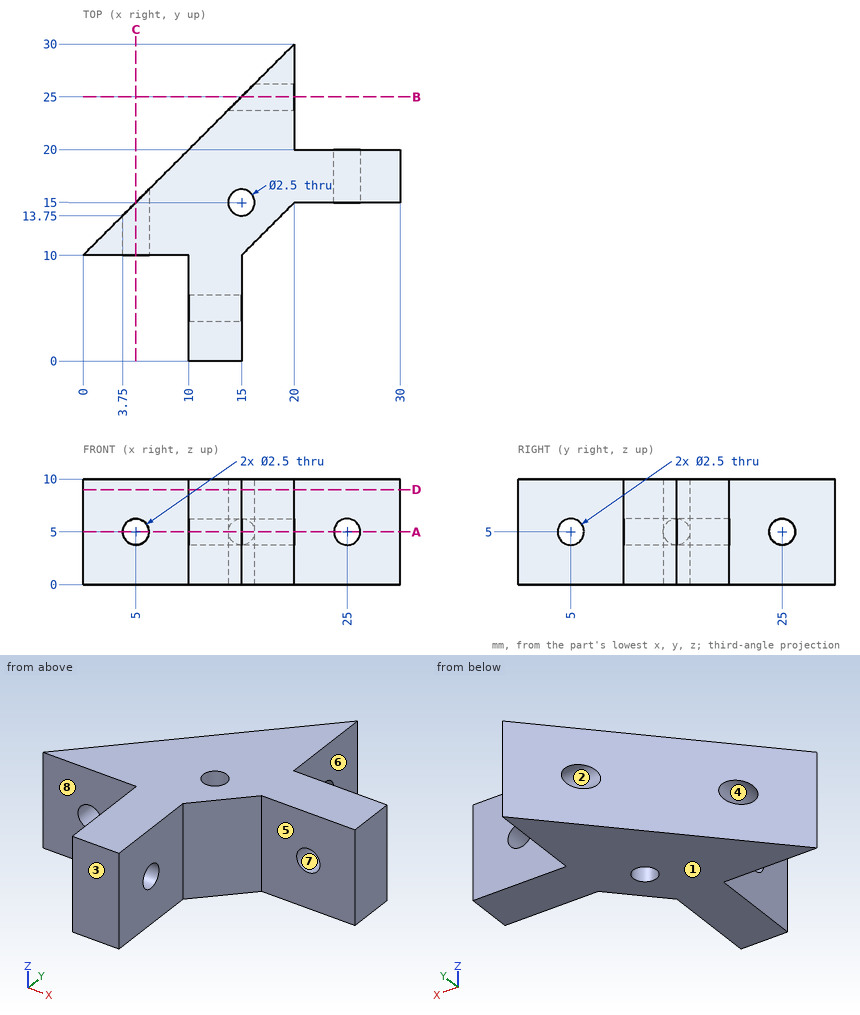
Part print with two shaded views. Sizes in mm from the minimum x, y, z corner. A direction names the side the tool comes from. Coordinates: 2 decimals unless noted, no trailing zeros. Write each loop counter-clockwise with the first axis right and the second up, starting at its lowest first coordinate (ties: lowest second). Pieces come first, ordered by that corner, then holes. Notation, with made-up numbers: (16.25, 55) - (63.25, 55) arc R12 cw to (63.25, 71) - close; hole circle Ø10 at (32.25, -18.75). An arc over 180 degrees is marked (long way). Put each result on its own line as item: value.
1. Band-saw the part on B-B (y = 25). Write the cut outline in (x, z).
Final values:
outline: (15, 0) - (20, 0) - (20, 3.75) - (15, 3.75) - close; (15, 6.25) - (20, 6.25) - (20, 10) - (15, 10) - close
2. Band-saw the part on C-C (x = 5). Write the cut outline in (y, z), then the cut area to 3 significant figures.
Final values:
outline: (10, 0) - (15, 0) - (15, 3.75) - (10, 3.75) - close; (10, 6.25) - (15, 6.25) - (15, 10) - (10, 10) - close
area: 37.5 mm²
3. Flat gauge pins, fed straight in: pin 1 Ø3 at (y, z) = (26.5, 6) entering from +X; pin 2 Ø5 at (x, z) = (25, 4) entering from -Y; pin 3 Ø6 at (x, z) = (20, 3) entering from -Y; pin 4 Ø6 at (x, y) = (4, 20) entering from +Z. Where does each tip first touch, or does it go through?
Final values:
pin 1: stops at x = 20
pin 2: stops at y = 15
pin 3: stops at y = 12
pin 4: passes through
4. Band-saw the part on A-A (z = 5). Write the cut outline in (x, y).
Final values:
outline: (0, 10) - (3.75, 10) - (3.75, 13.75) - close; (6.25, 10) - (10, 10) - (10, 6.25) - (15, 6.25) - (15, 10) - (20, 15) - (23.75, 15) - (23.75, 20) - (20, 20) - (20, 23.75) - (13.75, 23.75) - (6.25, 16.25) - close; (10, 0) - (15, 0) - (15, 3.75) - (10, 3.75) - close; (16.25, 26.25) - (20, 26.25) - (20, 30) - close; (26.25, 15) - (30, 15) - (30, 20) - (26.25, 20) - close; hole circle Ø2.5 at (15, 15)
5. Two-plate mould, pull along Z, no slides. Class the marked faces 1, 2, 3 and 4: +Z half, -Z half, draft (parallel to the pull), parting line (faces both ways), or undercut.
Final values:
face 1: -Z half
face 2: undercut
face 3: draft
face 4: undercut
6. Band-saw the part on D-D (z = 9). Write the cut outline in (x, y), then the cut area to 3 significant figures.
Final values:
outline: (0, 10) - (10, 10) - (10, 0) - (15, 0) - (15, 10) - (20, 15) - (30, 15) - (30, 20) - (20, 20) - (20, 30) - close; hole circle Ø2.5 at (15, 15)
area: 283 mm²
7. 3-axis set-ups, long thin cutter, end or side, ignore diameter. For the marked faces 5, 6, 7 and 8: which of +Z, -Z, +X, -X, +Y, -Y reach the whole face in a straight line?
Final values:
face 5: +Z, -Z, +X, -Y
face 6: +Z, -Z, +X, +Y
face 7: +Y, -Y
face 8: +Z, -Z, -X, -Y
8. Probe line 1 along Z through (x, y) = (25, 18.5); line 2 along Y through (x, z) = (13.95, 5); line 3 along Y through (x, z) = (13.9, 5). List the from-to ranges inside material, lowest first. Write a range as [from, to].
Final values:
line 1: z = [0, 3.75], [6.25, 10]
line 2: y = [0, 3.75], [6.25, 14.32], [15.68, 23.75]
line 3: y = [0, 3.75], [6.25, 14.41], [15.59, 23.75]
